```python
from build123d import *

# Parameters (mm, degrees)
SKETCH_1_R               = 25
EXTRUDE_2_DEPTH          = 170
SKETCH_2_R               = 3
CUT_EXTRUDE_1_DEPTH      = 10
PATTERN_CIRCULAR_1_COUNT = 4
MIRROR_1_OUTLINE_R       = 3
MIRROR_1_DEPTH           = 10
SKETCH_3_R               = 3
CUT_EXTRUDE_2_DEPTH      = 50


# Read off the part's stored shape, not the designer's step: 镜向1
with BuildPart() as part:
    # 草图1 → 凸台-拉伸2 (new body)
    with BuildSketch(Plane.XY):
        Circle(SKETCH_1_R)
    extrude(amount=EXTRUDE_2_DEPTH)

    # 草图2 → 切除-拉伸1 (cut)
    with BuildSketch(Plane.XY.offset(170)):
        with Locations((-18, 0)):
            Circle(SKETCH_2_R)
    cut_extrude_1 = extrude(amount=-CUT_EXTRUDE_1_DEPTH, mode=Mode.SUBTRACT)

    # 阵列(圆周)1: 切除-拉伸1 ×4 about axis
    pattern_circular_1_axis = Axis((0.262987013, 0, 0), (0, 0, 1))
    for i in range(1, PATTERN_CIRCULAR_1_COUNT):
        add(cut_extrude_1.rotate(pattern_circular_1_axis, i * 360 / PATTERN_CIRCULAR_1_COUNT), mode=Mode.SUBTRACT)

    # 镜向1 outline → 镜向1 (cut)
    with BuildSketch(Plane.XY):
        with Locations((-18, 0)):
            Circle(MIRROR_1_OUTLINE_R)
        with Locations((-0.016073909, 17.983926091)):
            Circle(MIRROR_1_OUTLINE_R)
        with Locations((17.967852182, 0)):
            Circle(MIRROR_1_OUTLINE_R)
        with Locations((-0.016073909, -17.983926091)):
            Circle(MIRROR_1_OUTLINE_R)
    extrude(amount=MIRROR_1_DEPTH, mode=Mode.SUBTRACT)

    # 草图3 → 切除-拉伸2 (cut)
    with BuildSketch(Plane(origin=(0, 0, 0), x_dir=(0, 0, -1), z_dir=(1, 0, 0))):
        with Locations((-85, 0)):
            Circle(SKETCH_3_R)
        with Locations((-85, 15)):
            Circle(SKETCH_3_R)
        with Locations((-85, -15)):
            Circle(SKETCH_3_R)
    extrude(amount=-CUT_EXTRUDE_2_DEPTH, mode=Mode.SUBTRACT)


solid = part.part
```
The listing builds one solid part. Answer for the finished solid, in the listing's coordinates (mm). A direction names the side the tool comes from. Round coordinates to 2 decimals unless told otherwise and drop trailing zeros. Loops run counter-clockwise (first coordinate to the right, second up) from the corner with the lowest first, then second, coordinate; pieces in that order, holes last. Notation, with made-up numbers: (-25, 27) -> (25, 27) arc R12 ccw to (25, 43) -> close; hole circle Ø3 at (61, -37). An arc over 180 degrees is marked (long way). Use one line per item in the form item = value.
1. A tool of negligible diameter and unlimited length cuts with its end or side. For faces 3 (the flat face through (0, -18, 160)), 4 (the cylindrical face through (-0.41, -15.01, 4.93)), 5 (the flat face through (0, 0, 85)), from which of +Z, -Z, +X, -X, +Y, -Y can it reach the whole face along a straight path? Write none if from no direction.
Answer key:
face_3 = +Z
face_4 = -Z
face_5 = -X
2. The part is cut by section B-B on z = 85. Determine the outline of the cut face in (x, y).
Answer key:
outline = (-24.82, -3) arc R25 ccw to (-21.93, -12) -> (0, -12) -> (0, -18) -> (-17.35, -18) arc R25 ccw (long way) to (-17.35, 18) -> (0, 18) -> (0, 12) -> (-21.93, 12) arc R25 ccw to (-24.82, 3) -> (0, 3) -> (0, -3) -> close
3. Flat-ended cylindrical pins translate along their axes: pin 1 Ø12 at (x, z) = (15.5, 82.5) entering from +Y; pin 2 Ø3 at (x, y) = (17.5, -1) entering from -Z; pin 3 Ø6 at (x, z) = (-3.5, 21.5) entering from +Y (3 decimals). Find the tip coordinate at first contact, or state that the pin passes through.
Answer key:
pin_1 = 23.12
pin_2 = 10
pin_3 = 24.995
4. For a pull along Y with two mould halves and no side action, classify faces 1 (the flat face through (0, 0, 170)), 2 (the cylindrical face through (-0.886, 15.492, 165.07)) as released by +Y, released by -Y, zero draft, split by the parting line, or undercut.
Answer key:
face_1 = zero draft
face_2 = undercut
5. The part is cut by section A-A on x = -17. Determine the outline of the cut face in (y, z).
Answer key:
outline = (-18.33, 0) -> (-2.83, 0) -> (-2.83, 10) -> (2.83, 10) -> (2.83, 0) -> (18.33, 0) -> (18.33, 170) -> (2.83, 170) -> (2.83, 160) -> (-2.83, 160) -> (-2.83, 170) -> (-18.33, 170) -> close; hole circle Ø6 at (-15, 85); hole circle Ø6 at (0, 85); hole circle Ø6 at (15, 85)
6. The part is cut by section C-C on y = 10.5. Determine the outline of the cut face in (x, z).
Answer key:
outline = (-22.69, 0) -> (22.69, 0) -> (22.69, 170) -> (-22.69, 170) -> close
7. Find the intervals of material crossed by probe 1 along Z at (x, y) = (-18.5, 0); probe 2 along Z at (x, y) = (-13, 15); probe 3 along Y at (x, z) = (-15, 85), in increasing order. Write a range as [from, to].
Answer key:
probe_1 = [10, 82], [88, 160]
probe_2 = [0, 82], [88, 170]
probe_3 = [-20, -18], [-12, -3], [3, 12], [18, 20]
8. The part is cut by section D-D on x = 9. Determine the outline of the cut face in (y, z).
Answer key:
outline = (-23.32, 0) -> (23.32, 0) -> (23.32, 170) -> (-23.32, 170) -> close
